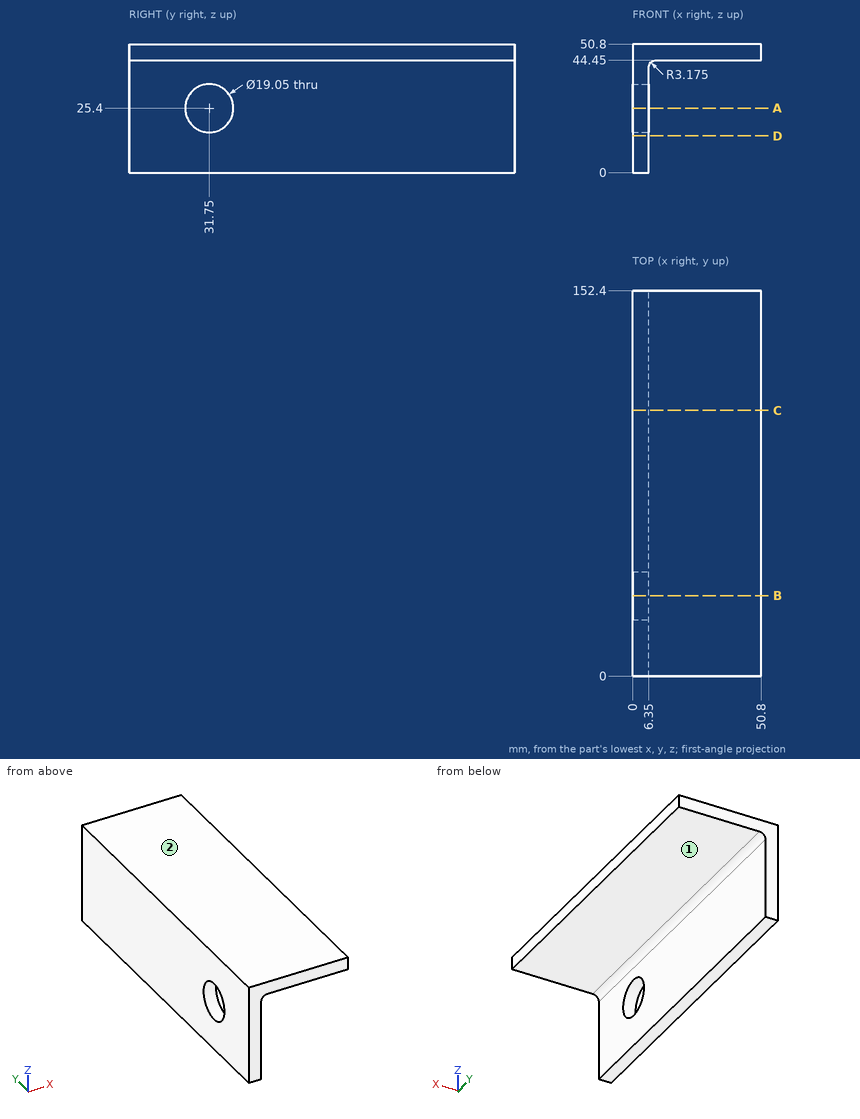
Could you check a few things on this drawing? It's one solid part, dimensions in mm from its lowest x, y, z. A direction names the side the tool comes from. Coordinates: 2 decimals unless noted, no trailing zeros. Loops run counter-clockwise (first coordinate to the right, second up) from the corner with the lowest first, then second, coordinate; pieces in that order, holes last. Notation, with made-up numbers: (74, -30.75) - (102, -30.75) arc R19 ccw to (102, 1.25) - close; hole circle Ø8 at (77.25, 71.25). An arc over 180 degrees is marked (long way). Answer as a JSON object with one key per item and string values. Group by question number.
Item 1: If we section it at D-D (z = 14.5): List the corners of the cut face in (x, y) for me.
Item 2: On a 3-axis mill with a long thin cutter (end or side, diameter ignored), from which of +Z, -Z, +X, -X, +Y, -Y can I reach the whole of each face in a straight line? I mean the marked faces 1 and 2. Say none if no direction works.
Item 3: If I drill on L1, parallel to Y at x = 4, z = 25; L2, parallel to Z at x = 38, y = 76; L3, parallel to X at y = 99, z = 17, over which ranges is the centre line in solid material (lowest first)? Write a range as from..to.
Item 4: For pin 1 (20.5 mm diameter, centred on y = 45.5, z = 24, fed in from +X); pin 2 (6 mm diameter, centred on x = 45, y = 82.5, fed in from -Z), each with a flat end and sliding along its axis, tell me the tip position at first contact or that it passes through.
Item 5: If we section it at C-C (y = 105): List the corners of the cut face in (x, z) for me (3 decimals).
Item 6: If we section it at A-A (z = 25.4): List the corners of the cut face in (x, y) for me (3 decimals), plus the area to 3 significant figures.
Item 7: If we section it at B-B (y = 31.75): List the corners of the cut face in (x, z) for me (3 decimals).
Returned:
{
 "1": {"outline": "(0, 0) - (6.35, 0) - (6.35, 152.4) - (0, 152.4) - close"},
 "2": {"face 1": "-Z, +X, +Y, -Y", "face 2": "+Z, +X, -X, +Y, -Y"},
 "3": {"L1": "y = 0..22.23, 41.27..152.4", "L2": "z = 44.45..50.8", "L3": "x = 0..6.35"},
 "4": {"pin 1": "stops at x = 6.35", "pin 2": "stops at z = 44.45"},
 "5": {"outline": "(0, 0) - (6.35, 0) - (6.35, 41.275) arc R3.175 cw to (9.525, 44.45) - (50.8, 44.45) - (50.8, 50.8) - (0, 50.8) - close"},
 "6": {"outline": "(0, 0) - (6.35, 0) - (6.35, 22.225) - (0, 22.225) - close; (0, 41.275) - (6.35, 41.275) - (6.35, 152.4) - (0, 152.4) - close", "area": "847 mm²"},
 "7": {"outline": "(0, 0) - (6.35, 0) - (6.35, 15.875) - (0, 15.875) - close; (0, 34.925) - (6.35, 34.925) - (6.35, 41.275) arc R3.175 cw to (9.525, 44.45) - (50.8, 44.45) - (50.8, 50.8) - (0, 50.8) - close"}
}
